Input: part model. Units: mm. Frame: model coordinates. A direction names the side the tool comes from. Coordinates: 2 decimals unless noted, no trailing zeros. Order: outer loops, then holes, each group sorted by start corner. A loop starts at its lowest first (then second) coordinate and runs counter-clockwise, first axis right, second up. Notation, with made-up numbers: (-7, 18) - (2, 18) arc R29 ccw to (2, 47) - close; hole circle Ø8 at (4.25, -4). An arc over 180 degrees is marked (long way). One line per question, with ' | ' between items.
from build123d import *

# Parameters (mm, degrees)
SKETCH2_R           = 4.7625
BOSS_EXTRUDE1_DEPTH = 65.1002
CUT_EXTRUDE1_DEPTH  = 3.175
CHAMFER1_SIZE       = 0.508


with BuildPart() as part:
    # Sketch2 → Boss-Extrude1 (new body)
    with BuildSketch(Plane.XY):
        Circle(SKETCH2_R)
    extrude(amount=BOSS_EXTRUDE1_DEPTH)

    # Sketch3 → Cut-Extrude1 (cut)
    with BuildSketch(Plane.XY.offset(65.1002)):
        Polygon((4.7625, 0), (4.7625, 1.27), (-4.7625, 1.27), (-4.7625, 0), (-4.7625, -1.27), (4.7625, -1.27), align=None)
    extrude(amount=-CUT_EXTRUDE1_DEPTH, mode=Mode.SUBTRACT)

    # Chamfer1
    chamfer1_edges = [part.edges().sort_by_distance(p)[0] for p in [
        (-4.7625, 0, 0),
        (0, 4.7625, 65.1002),
        (0, -4.7625, 65.1002),
    ]]
    chamfer(chamfer1_edges, length=CHAMFER1_SIZE)


solid = part.part
Item 1: Ray query, line 1 (X direction, y = -2.5, z = 20.5); line 2 (X direction, y = 0.25, z = 5); line 3 (Z direction, x = -3.25, y = -1). Return the intervals inside material, ascending.
Data:
line 1: -4.05 to 4.05 | line 2: -4.76 to 4.76 | line 3: 0 to 61.93
Item 2: Draft query along Y for faces 3 (the face through (0, 1.27, 64)), 4 (the face through (0, 2, 65.1)), 5 (the face through (0.08, 4.391, 64.963)), 6 (the face through (0, 0, 61.925)). Return one class per face: released by +Y, released by -Y, zero draft, split by the parting line, or undercut.
Data:
face 3: undercut | face 4: zero draft | face 5: released by +Y | face 6: undercut
Item 3: Contact query for flat-ended pins moving along their axis: P1, Ø4, axis at x = 3.5, y = -2.5, coming from the -Z side; P2, Ø2, axis at x = 3.5, z = 51.5, coming from the -Y side; P3, Ø1.6, axis at x = -1, z = 63.5, coming from the +Y side. Output: stop coordinate, or through.
Data:
P1: z = 0 | P2: y = -4.05 | P3: y = 4.76
Item 4: Section A-A on y = 0. Return the cut outline in (x, z).
Data:
outline: (-4.76, 0.51) - (-4.25, 0) - (4.25, 0) - (4.76, 0.51) - (4.76, 61.93) - (-4.76, 61.93) - close
Item 5: Access query for faces 1 (the face through (0, -1.27, 64)), 2 (the face through (0, 0, 0)). Directions: +Z, -Z, +X, -X, +Y, -Y. A direction counts if a zero-diameter tool reaches every point of the face in a straight line with its end or side. Return the directions, or none.
Data:
face 1: +Z, +X, -X | face 2: -Z, +X, -X, +Y, -Y
Item 6: Section B-B on z = 25.5. Return the cut outline in (x, y) (1 decimal), and give its area (3 significant figures).
Data:
outline: circle Ø9.5 at (0, 0) | area: 71.3 mm^2
